from build123d import *

# Parameters (mm, degrees)
BOSS_EXTRUDE1_DEPTH = 1.5875
SKETCH8_R           = 6.35
CUT_EXTRUDE1_DEPTH  = 5.08


with BuildPart() as part:
    # Sketch3 → Boss-Extrude1 (new body, symmetric)
    with BuildSketch(Plane(origin=(0, 0, 0), x_dir=(1, 0, 0), z_dir=(0, 1, 0))):
        Polygon((-279.4, 95.25), (-139.7, 95.25), (-120.65, 133.35), (133.35, 133.35), (152.4, 95.25), (279.4, 95.25), (279.4, -95.25), (152.4, -95.25), (133.35, -133.35), (-120.65, -133.35), (-139.7, -95.25), (-279.4, -95.25), align=None)
    extrude(amount=BOSS_EXTRUDE1_DEPTH, both=True)

    # Sketch8 → Cut-Extrude1 (cut)
    with BuildSketch(Plane(origin=(0, 1.5875, 0), x_dir=(1, 0, 0), z_dir=(0, 1, 0))):
        with Locations((-241.3, 0)):
            Circle(SKETCH8_R)
    extrude(amount=-CUT_EXTRUDE1_DEPTH, mode=Mode.SUBTRACT)


solid = part.part
Input: part model. Units: mm. Frame: model coordinates. Give positions to 0.01 mm unless a question says otherwise; leave off trailing zeros. Write each loop counter-clockwise with the first axis right and the second up, starting at its lowest first coordinate (ties: lowest second). Pieces come first, ordered by that corner, then holes. Notation, with made-up numbers: M -31,-36.5 L -22,-36.5 A22 ccw -22,-26.5 Z; hole C 58.25,-26 d11. An arc over 180 degrees is marked long. Use one line per item in the form item = value.
1. Cut plane C-C on y = 0.3. Return loops of the section in (x, z), and give its area (3 significant figures).
Outcome:
outline = M -279.4,-95.25 L -139.7,-95.25 L -120.65,-133.35 L 133.35,-133.35 L 152.4,-95.25 L 279.4,-95.25 L 279.4,95.25 L 152.4,95.25 L 133.35,133.35 L -120.65,133.35 L -139.7,95.25 L -279.4,95.25 Z; hole C -241.3,0 d12.7
area = 127,000 mm²
2. Mould query, pull axis Z, two halves, no side actions, for faces 1 (the face through (143.01, 0.02, 114.03)), 2 (the face through (-247.644, 0.022, -0.279)), 3 (the face through (142.74, 0.02, -114.57)). Classes: released by +Z, released by -Z, zero draft, split by the parting line, or undercut.
Outcome:
face_1 = released by +Z
face_2 = undercut
face_3 = released by -Z
3. Cut plane D-D on x = 171. Return loops of the section in (y, z), and give its area (3 significant figures).
Outcome:
outline = M -1.59,-95.25 L 1.59,-95.25 L 1.59,95.25 L -1.59,95.25 Z
area = 605 mm²
4. Cut plane B-B on x = -241.3. Return loops of the section in (y, z), and give its area (3 significant figures).
Outcome:
outline = M -1.59,-95.25 L 1.59,-95.25 L 1.59,-6.35 L -1.59,-6.35 Z; M -1.59,6.35 L 1.59,6.35 L 1.59,95.25 L -1.59,95.25 Z
area = 565 mm²
5. Cut plane A-A on z = 0. Return loops of the section in (x, y), and give its area (3 significant figures).
Outcome:
outline = M -279.4,-1.59 L -247.65,-1.59 L -247.65,1.59 L -279.4,1.59 Z; M -234.95,-1.59 L 279.4,-1.59 L 279.4,1.59 L -234.95,1.59 Z
area = 1,730 mm²
6. Ray query, L1, parallel to X at y = 0.7, z = 0; L2, parallel to Z at x = -241.3, y = 0.8; L3, parallel to X at y = 1, z = -113 (3 decimals). Return the intervals inside material, ascending.
Outcome:
L1 = -279.4 to -247.65, -234.95 to 279.4
L2 = -95.25 to -6.35, 6.35 to 95.25
L3 = -130.825 to 143.525
